Check sheet for the modelled part. Datum: model origin and axes. Units: mm. Face numbers are marked on the shaded views. A direction names the side the tool comes from. Give positions to 0.01 mm unless a question says otherwise; leave off trailing zeros. Write each loop counter-clockwise with the first axis right and the second up, starting at its lowest first coordinate (ties: lowest second). Pieces come first, ordered by that corner, then holes. Notation, with made-up numbers: (-27.5, -24.5) - (-4.5, -24.5) arc R23 ccw to (-4.5, 11.5) - close; hole circle Ø5 at (3.25, 34). An arc over 180 degrees is marked (long way). Return JSON: item names as keys, results as strings. Group by question number.
```python
from build123d import *

# Parameters (mm, degrees)
BOSS_EXTRUDE2_DEPTH = 31.75
CUT_EXTRUDE1_REACH  = 115.77
SKETCH2_R           = 3.175
CUT_EXTRUDE2_REACH  = 115.77
SKETCH3_R           = 3.175
FILLET2_R           = 2.54


with BuildPart() as part:
    # Sketch1 → Boss-Extrude2 (new, symmetric)
    with BuildSketch(Plane.XY):
        Polygon((0, 0), (0, 88.9), (6.35, 88.9), (6.35, 6.35), (63.5, 6.35), (63.5, 0), align=None)
    extrude(amount=BOSS_EXTRUDE2_DEPTH, both=True)

    # Sketch2 → Cut-Extrude1 (cut, up to next)
    with BuildSketch(Plane.ZY, mode=Mode.PRIVATE) as cut_extrude1_sk1:
        with Locations((0, 63.5)):
            Circle(SKETCH2_R)
    cut_extrude1_tool1 = extrude(cut_extrude1_sk1.sketch, amount=-CUT_EXTRUDE1_REACH, mode=Mode.PRIVATE) & part.part
    # Sketch2 → Cut-Extrude1 (cut, up to next)
    with BuildSketch(Plane.ZY, mode=Mode.PRIVATE) as cut_extrude1_sk2:
        with Locations((0, 38.1)):
            Circle(SKETCH2_R)
    cut_extrude1_tool2 = extrude(cut_extrude1_sk2.sketch, amount=-CUT_EXTRUDE1_REACH, mode=Mode.PRIVATE) & part.part
    add(cut_extrude1_tool1.solids().sort_by_distance((0, 63.5, 0))[0], mode=Mode.SUBTRACT)
    add(cut_extrude1_tool2.solids().sort_by_distance((0, 38.1, 0))[0], mode=Mode.SUBTRACT)

    # Sketch3 → Cut-Extrude2 (cut, up to next)
    with BuildSketch(Plane.XZ, mode=Mode.PRIVATE) as cut_extrude2_sk1:
        with Locations((25.4, 0)):
            Circle(SKETCH3_R)
    cut_extrude2_tool1 = extrude(cut_extrude2_sk1.sketch, amount=-CUT_EXTRUDE2_REACH, mode=Mode.PRIVATE) & part.part
    # Sketch3 → Cut-Extrude2 (cut, up to next)
    with BuildSketch(Plane.XZ, mode=Mode.PRIVATE) as cut_extrude2_sk2:
        with Locations((50.8, 0)):
            Circle(SKETCH3_R)
    cut_extrude2_tool2 = extrude(cut_extrude2_sk2.sketch, amount=-CUT_EXTRUDE2_REACH, mode=Mode.PRIVATE) & part.part
    add(cut_extrude2_tool1.solids().sort_by_distance((25.4, 0, 0))[0], mode=Mode.SUBTRACT)
    add(cut_extrude2_tool2.solids().sort_by_distance((50.8, 0, 0))[0], mode=Mode.SUBTRACT)

    # Fillet2
    fillet2_edges = [part.edges().sort_by_distance(p)[0] for p in [
        (6.35, 6.35, 0),
    ]]
    fillet(fillet2_edges, radius=FILLET2_R)


solid = part.part
```
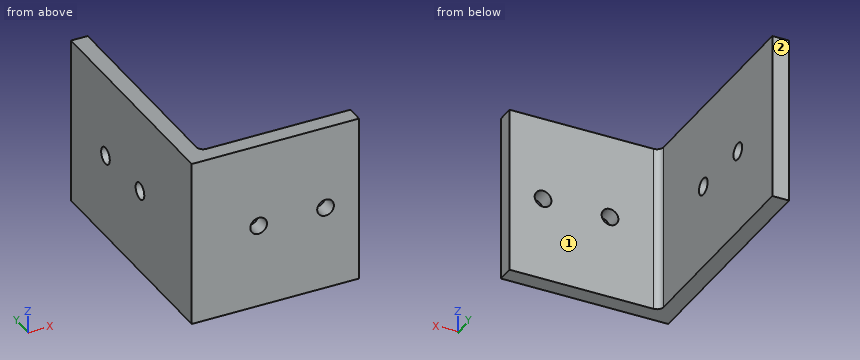
Item 1: Access from +Z, -Z, +X, -X, +Y, -Y to the whole of each face (thin tool, end or side, straight path). Record for the marked faces 1 and 2.
Item 2: Depth check by flat-ended pin: pin 1 (5 mm diameter, centred on x = 50.8, z = 0, fed in from +Y); pin 2 (6 mm diameter, centred on x = 50.5, z = 13, fed in from +Y). Enter the tip coordinate at first touch or a pass-through.
Item 3: Section check D-D on z = -13. Record the cut outline in (x, y).
Item 4: Section check C-C on z = 0. Record the cut outline in (x, y) (3 decimals).
Item 5: Section check A-A on y = 63.5. Record the cut outline in (x, z) (3 decimals), plus the area to 3 significant figures.
Item 6: Material ranges on line 1 along Y through (x, z) = (2.25, 0) (3 decimals); line 2 along X through (y, z) = (46, 12), recorded low to high. Write a range as from..to.
Reply:
{
 "1": {"face 1": "+Z, -Z, +X, +Y", "face 2": "+Z, -Z, +X, -X, +Y"},
 "2": {"pin 1": "through", "pin 2": "y = 6.35"},
 "3": {"outline": "(0, 0) - (63.5, 0) - (63.5, 6.35) - (8.89, 6.35) arc R2.54 cw to (6.35, 8.89) - (6.35, 88.9) - (0, 88.9) - close"},
 "4": {"outline": "(0, 0) - (22.225, 0) - (22.225, 6.35) - (8.89, 6.35) arc R2.54 cw to (6.35, 8.89) - (6.35, 34.925) - (0, 34.925) - close; (0, 41.275) - (6.35, 41.275) - (6.35, 60.325) - (0, 60.325) - close; (0, 66.675) - (6.35, 66.675) - (6.35, 88.9) - (0, 88.9) - close; (28.575, 0) - (47.625, 0) - (47.625, 6.35) - (28.575, 6.35) - close; (53.975, 0) - (63.5, 0) - (63.5, 6.35) - (53.975, 6.35) - close"},
 "5": {"outline": "(0, -31.75) - (6.35, -31.75) - (6.35, -3.175) - (0, -3.175) - close; (0, 3.175) - (6.35, 3.175) - (6.35, 31.75) - (0, 31.75) - close", "area": "363 mm²"},
 "6": {"line 1": "0..34.925, 41.275..60.325, 66.675..88.9", "line 2": "0..6.35"}
}
